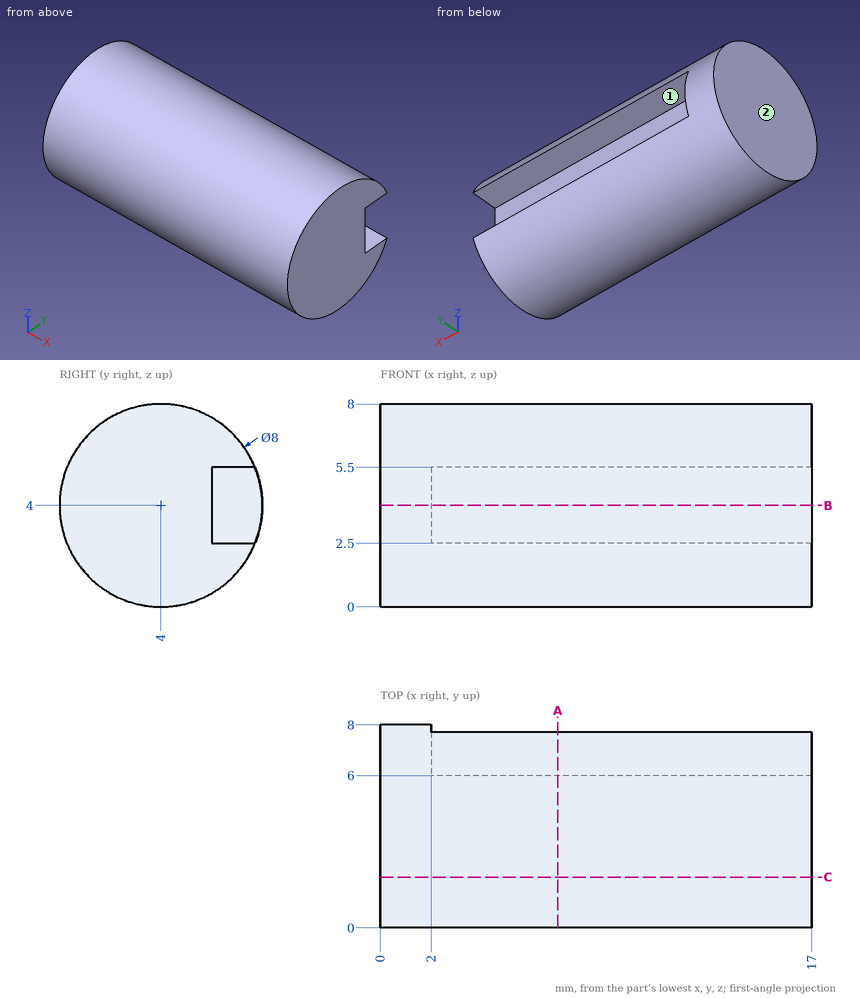
Geometry check sheet. Reference: drawing and pictorial views, mm from the part's lowest x, y, z. A direction names the side the tool comes from. Round coordinates to 2 decimals unless told otherwise and drop trailing zeros. Order: outer loops, then holes, each group sorted by start corner. A loop starts at its lowest first (then second) coordinate and runs counter-clockwise, first axis right, second up.
Q1. Set-up check for the marked faces 1 and 2: record each of +Z, -Z, +X, -X, +Y, -Y from which the full face is reachable in a straight line by a thin tool's end or side.
Filled sheet:
face 1: +X, +Y
face 2: +Z, -Z, -X, +Y, -Y
Q2. Depth check by flat-ended pin: P1, Ø0.5, axis at x = 9.5, y = 7, coming from the -Z side; P2, Ø0.6, axis at y = 6.5, z = 4.5, coming from the +X side; P3, Ø0.9, axis at x = 12, z = 4.5, coming from the +Y side. Enter the tip coordinate at first touch or a pass-through.
Filled sheet:
P1: stops at z = 1.1
P2: stops at x = 2
P3: stops at y = 6
Q3. Cross-section at A-A, the plane x = 7. Enter the section's corners in (y, z), plus the area to 3 significant figures.
Filled sheet:
outline: (6, 2.5) - (6, 5.5) - (7.71, 5.5) arc R4 ccw (long way) to (7.71, 2.5) - close
area: 44.6 mm2
Q4. Scan lines: L1, parallel to Z at x = 11.5, y = 7.25; L2, parallel to Y at x = 5.25, z = 6.25; L3, parallel to Y at x = 8, z = 5. Record each from-to range of solid material in increasing order.
Filled sheet:
L1: z = 1.67 to 2.5, 5.5 to 6.33
L2: y = 0.69 to 7.31
L3: y = 0.13 to 6
Q5. Cross-section at B-B, the plane z = 4. Enter the section's corners in (x, y), plus the area to 3 significant figures.
Filled sheet:
outline: (0, 0) - (17, 0) - (17, 6) - (2, 6) - (2, 8) - (0, 8) - close
area: 106 mm2
Q6. Cross-section at C-C, the plane y = 2. Enter the section's corners in (x, z).
Filled sheet:
outline: (0, 0.54) - (17, 0.54) - (17, 7.46) - (0, 7.46) - close
